The listing builds one solid part. Answer for the finished solid, in the listing's coordinates (mm). A direction names the side the tool comes from. Give positions to 0.01 mm unless a question says otherwise; leave off trailing zeros. Loops run counter-clockwise (first coordinate to the right, second up) from the corner with the lowest first, then second, coordinate; pieces in that order, holes last.
Item 1: The mould has two halves that part along X. Classify faces 1 (the face through (5, 5, 15)), 2 (the face through (17.582, -10.251, 7.395)), 3 (the face through (-2.46, -1.51, 2.46)), 4 (the face through (-4.632, -1.453, 17.535)): pulls with the +X half, pulls with the -X half, needs draft (parallel to the pull), parting line crosses it, or undercut.
Item 2: Section A-A, the plane z = 2 is taken. Give the vertices of the cut face in (x, y).
Item 3: Consider line 1 along Z through (x, y) = (-19, 6); line 2 along Y through (x, z) = (10.5, 8.25); line 3 along Y through (x, z) = (-9.5, 8). Determine where each line is inside the solid, lowest interval first.
Item 4: Each of these flat-tipped pins is pushed along its axis until it touches: pin 1 Ø1.5 at (x, z) = (-1.5, 17) entering from -Y; pin 2 Ø1 at (x, z) = (-13, 6) entering from -Y; pin 3 Ø2 at (x, z) = (15, 13) entering from -Y. Where does it stop, or does it pass through?
Item 5: Section D-D, the plane x = 19 is taken. Give the vertices of the cut face in (y, z).
Item 6: Section B-B, the plane y = 4 is taken. Give the vertices of the cut face in (x, z), and give its area (3 significant figures).
Item 7: A tool of negligible diameter and unlimited length cuts with its end or side. For faces 5 (the face through (-2.81, 3.96, 17.54)), 6 (the face through (0, -4.854, 18)), 7 (the face through (4.6, -1.55, 17.54)), 8 (the face through (0, -1, 5)), 9 (the face through (2.89, 3.9, 17.54)), from which of +Z, -Z, +X, -X, +Y, -Y can it reach the whole face along a straight path? Write none if from no direction.
Item 8: Section C-C, the plane z = 9.5 is taken. Give the vertices of the cut face in (x, y), and give its area (3 significant figures).
from build123d import *

# Parameters (mm, degrees)
F1_DEPTH = 15
F3_DEPTH = 5
F5_DEPTH = 5


with BuildPart() as f1:
    # F0 (on Top) → F1 (new body)
    with BuildSketch(Plane.XY):
        Polygon((-11.82836, 20.306155), (-23.499825, -0.090583), (-11.671466, -20.396737), (11.82836, -20.306155), (23.499825, 0.090583), (11.671466, 20.396737), align=None)
    extrude(amount=F1_DEPTH)

    # F2 (on face) → F3 (join, symmetric)
    with BuildSketch(Plane.XY.offset(15)):
        Polygon((-3.526712, -4.854102), (3.526712, -4.854102), (5.706339, 1.854102), (0, 6), (-5.706339, 1.854102), align=None)
    extrude(amount=F3_DEPTH, both=True)

    # F4 (on face) → F5 (cut)
    with BuildSketch(Plane(origin=(0, 0, 0), x_dir=(1, 0, 0), z_dir=(0, 0, -1))):
        Polygon((-5.01109, -2.867457), (4.988836, -2.906003), (0.022254, 5.77346), align=None)
    extrude(amount=-F5_DEPTH, mode=Mode.SUBTRACT)


solid = f1.part
Worked answers:
1. face 1: needs draft
1. face 2: pulls with the +X half
1. face 3: undercut
1. face 4: pulls with the -X half
2. outline: (-23.5, -0.09) - (-11.67, -20.4) - (11.83, -20.31) - (23.5, 0.09) - (11.67, 20.4) - (-11.83, 20.31) - close; hole (-5.01, 2.87) - (0.02, -5.77) - (4.99, 2.91) - close
3. line 1: z = 0 to 15
3. line 2: y = -20.31 to 20.39
3. line 3: y = -20.39 to 20.32
4. pin 1: stops at y = -4.85
4. pin 2: stops at y = -18.97
4. pin 3: stops at y = -16.51
5. outline: (-7.77, 0) - (7.82, 0) - (7.82, 15) - (-7.77, 15) - close
6. outline: (-21.16, 0) - (21.22, 0) - (21.22, 15) - (2.75, 15) - (2.75, 20) - (-2.75, 20) - (-2.75, 15) - (-21.16, 15) - close
6. area: 663 mm2
7. face 5: +Z, -X, +Y
7. face 6: +Z, +X, -X, -Y
7. face 7: +Z, +X, -Y
7. face 8: -Z
7. face 9: +Z, +X, +Y
8. outline: (-23.5, -0.09) - (-11.67, -20.4) - (11.83, -20.31) - (23.5, 0.09) - (11.67, 20.4) - (-11.83, 20.31) - close
8. area: 1,430 mm2
